Work out the finished part from the listing and answer in its coordinate system (mm). A direction names the side the tool comes from. Give positions to 0.01 mm unless a question says otherwise; leave off trailing zeros. Order: outer loops, then holes, each group sorted by start corner. A loop starts at its lowest first (then second) coordinate and runs counter-clockwise, first axis right, second up.
Autodesk Fusion 360 part; units mm, degrees
sketch "スケッチ1" plane through (0, 0, 0) normal (0, 0, 1) x (1, 0, 0)
  line L0 (-86.5, -163) -> (-3.5, -163)
  line L1 (86.5, 45) -> (86.5, 155)
  line L2 (-3.5, 163) -> (-86.5, 163)
  line L3 (-86.5, 163) -> (-86.5, -163)
  line L4 (-86.5, -163) -> (82.2546, 155) construction
  line L5 (39.184, -73.838) -> (-86.5, 163) construction
  line L6 (-3.5, 163) -> (-3.5, 155)
  line L7 (-3.5, 155) -> (86.5, 155)
  line L8 (-86.5, -163) -> (-3.5, -163) construction
  line L9 (86.5, 25) -> (-3.5, -163)
  line L10 (86.5, 25) -> (-3.5, 25)
  line L11 (-3.5, 25) -> (-3.5, 45)
  line L12 (-3.5, 45) -> (86.5, 45)
  dimension "d5" = 83
  dimension "d7" = 90
  dimension "d8" = 20
extrude "押し出し1" add sketch "スケッチ1" along normal blind 6
chamfer "面取り1" distance 30 angle 45 2 edges at (-86.5, -163, 3) (-86.5, 163, 3)
sketch "スケッチ2" plane through (0, 0, 6) normal (0, 0, 1) x (-1, 0, 0)
  line L0 (56.5, -163) -> (86.5, -133)
  line L1 (86.5, -133) -> (86.5, 133)
  line L2 (86.5, 133) -> (56.5, 163)
  line L3 (56.5, 163) -> (3.5, 163)
  line L4 (3.5, 163) -> (-86.5, -25)
  line L5 (-86.5, -25) -> (3.5, -25)
  line L6 (3.5, -25) -> (3.5, -45)
  line L7 (3.5, -45) -> (-86.5, -45)
  line L8 (-86.5, -45) -> (-86.5, -155)
  line L9 (-86.5, -155) -> (3.5, -155)
  line L10 (3.5, -155) -> (3.5, -163)
  line L11 (3.5, -163) -> (56.5, -163)
  line L12 (-86.5, -155) -> (-46.5, -155) construction
  line L13 (-46.5, -155) -> (-46.5, -125) construction
  line L14 (-46.5, -125) -> (-86.5, -125) construction
  line L15 (-86.5, -125) -> (-86.5, -155) construction
  line L16 (-46.5, -125) -> (-46.5, -75) construction
  point P0 (-46.5, -125)
  point P1 (-46.5, -75)
  dimension "d12" = 40
  dimension "d13" = 30
  dimension "d14" = 50
hole "穴1" at (46.5, 125, 6) at (46.5, 75, 6) direction (0, 0, -1) diameter 18 end through all
equation "d5 = 30 mm + 53 mm"
1. The part is cut by section D-D (x = 46.5). Write down the section's boundary in (y, z), then the cut area to 3 significant figures.
Findings below:
outline: (-58.56, 0) - (25, 0) - (25, 6) - (-58.56, 6) - close; (45, 0) - (66, 0) - (66, 6) - (45, 6) - close; (84, 0) - (116, 0) - (116, 6) - (84, 6) - close; (134, 0) - (155, 0) - (155, 6) - (134, 6) - close
area: 945 mm2
2. Straight lines are drawn through the part: probe 1 along X at (y, z) = (125, 4.2); probe 2 along Y at (x, z) = (46.5, 4.6); probe 3 along Y at (x, z) = (48, 0.5). For each, find the intervals that lie inside material, in ascending order.
Findings below:
probe 1: x = -86.5 to 37.5, 55.5 to 86.5
probe 2: y = -58.56 to 25, 45 to 66, 84 to 116, 134 to 155
probe 3: y = -55.42 to 25, 45 to 66.13, 83.87 to 116.13, 133.87 to 155
3. The part is cut by section A-A (y = 75). Write down the section's boundary in (x, z).
Findings below:
outline: (-86.5, 0) - (37.5, 0) - (37.5, 6) - (-86.5, 6) - close; (55.5, 0) - (86.5, 0) - (86.5, 6) - (55.5, 6) - close
4. The part is cut by section B-B (z = 4.75). Write down the section's boundary in (x, y), then the cut area to 3 significant figures.
Findings below:
outline: (-86.5, -133) - (-56.5, -163) - (-3.5, -163) - (86.5, 25) - (-3.5, 25) - (-3.5, 45) - (86.5, 45) - (86.5, 155) - (-3.5, 155) - (-3.5, 163) - (-56.5, 163) - (-86.5, 133) - close; hole circle Ø18 at (46.5, 75); hole circle Ø18 at (46.5, 125)
area: 44,000 mm2
5. The mould has two halves that part along Y. Classify faces 4 (the face through (41, 45, 3)), 5 (the face through (-30, -163, 3)), 6 (the face through (-71.3, 148.2, 3)): pulls with the +Y half, pulls with the -Y half, needs draft (parallel to the pull), parting line crosses it, or undercut.
Findings below:
face 4: undercut
face 5: pulls with the -Y half
face 6: pulls with the +Y half
6. Given P1, Ø10, axis at x = -68, y = 75.5, coming from the -Z side; P2, Ø1.8, axis at x = 36, z = 2.5, coming from the -Y side; P3, Ø3, axis at x = 40.5, z = 2, coming from the +Y side; P4, Ø2, axis at y = -45, z = 1, coming from the +X side, each flat-ended and moving along its own axis, determine where each tip first touches the part or whether it passes through.
Findings below:
P1: stops at z = 0
P2: stops at y = -82.37
P3: stops at y = 155
P4: stops at x = 53.47
7. Which of the six approach directions +Z, -Z, +X, -X, +Y, -Y give full straight-line access (tool end or side, diameter ignored) to faces 1 (the face through (42, 25, 3)), 2 (the face through (-3.5, 159, 3)), 3 (the face through (38.91, 120.16, 2.96))?
Findings below:
face 1: +Z, -Z, +X
face 2: +Z, -Z, +X, +Y
face 3: +Z, -Z
8. The part is cut by section C-C (x = 4.5). Write down the section's boundary in (y, z).
Findings below:
outline: (-146.29, 0) - (25, 0) - (25, 6) - (-146.29, 6) - close; (45, 0) - (155, 0) - (155, 6) - (45, 6) - close
